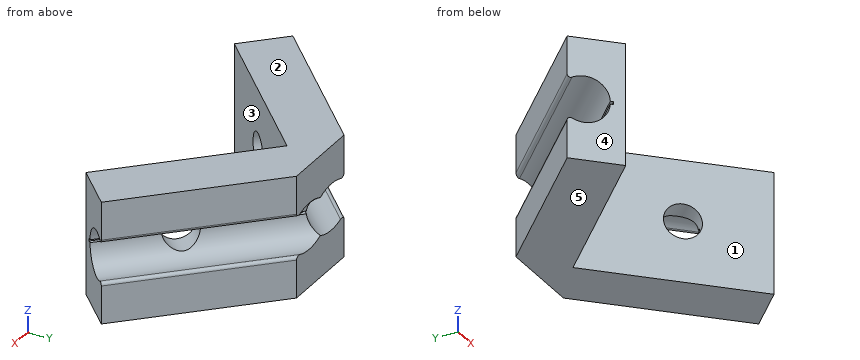
Autodesk Inventor part; units mm, degrees
ref_plane "Plano de trabajo1" through (0, 0, 0) normal (1, 0, 0) x (0, 0, -1)
ref_plane "Plano de trabajo2" through (28.2132, -15.4853, -21) normal (0.7071, 0.7071, 0) x (-0.7071, 0.7071, 0)
ref_plane "Plano de trabajo3" through (0, 0, -10.5) normal (0, 0, 1) x (1, 0, 0)
sketch "Sketch1" plane through (0, 0, 0) normal (0, 0, 1) x (1, 0, 0)
  line L0 (-7, 5.7279) -> (7, 5.7279)
  line L1 (-7, 5.7279) -> (-28.2132, -15.4853)
  line L2 (-28.2132, -15.4853) -> (-21.8492, -21.8492)
  line L3 (0, 0) -> (-21.8492, -21.8492)
  line L4 (7, 5.7279) -> (28.2132, -15.4853)
  line L5 (28.2132, -15.4853) -> (21.8492, -21.8492)
  line L6 (0, 0) -> (21.8492, -21.8492)
  line L7 (0, 15.5718) -> (0, -18.5373) construction
  dimension "d112" = 30
  dimension "d204" = 7
  dimension "d205" = 7
  dimension "d207" = 30
  dimension "d208" = 45
  dimension "d209" = 45
  dimension "d210" = 9
  dimension "d211" = 9
extrude "Extrusion1" add sketch "Sketch1" against normal blind 21
ref_plane "Plano de trabajo1" through (0, 0, 0) normal (1, 0, 0) x (0, 0, -1)
ref_plane "Plano de trabajo2" through (28.2132, -15.4853, -21) normal (0.7071, 0.7071, 0) x (-0.7071, 0.7071, 0)
sketch "Boceto2" plane through (28.2132, -15.4853, 0) normal (0.7071, -0.7071, 0) x (-0.7071, -0.7071, 0)
  line L0 (-3.8291, 10.5) -> (9.1738, 10.5) construction
  line L1 (0, 7.5) -> (0, 13.5)
  arc A0 (0, 7.5) -> (6.6379, 10.25) centre (2.6458, 10.5) ccw
  arc A1 (6.6379, 10.75) -> (0, 13.5) centre (2.6458, 10.5) ccw
  line L2 (0, 21) -> (9, 21)
  line L3 (9, 0) -> (0, 0)
  line L4 (7.1379, 10.75) -> (7.1379, 10.25)
  line L5 (7.1379, 10.25) -> (6.6379, 10.25)
  line L6 (7.1379, 10.75) -> (6.6379, 10.75)
  point P0 (0.9314, 0)
  dimension "d163" = 6
  dimension "d164" = 3
  dimension "d167" = 4
  dimension "d171" = 10.5
  dimension "d172" = 10.5
  dimension "d179" = 0.25
  dimension "d180" = 0.5
  dimension "d181" = 0.5
extrude "Extrusión2" cut sketch "Boceto2" against normal up to surface surface through (0, 0, 0) normal (1, 0, 0)
mirror "Simetría1" about plane through (0, 0, 0) normal (1, 0, 0) of "Extrusión2"
fillet "Empalme1" radius 0.5 4 edges at (17.6066, -4.8787, -7.5) (17.6066, -4.8787, -13.5) (-17.6066, -4.8787, -13.5) (-17.6066, -4.8787, -7.5)
sketch "Boceto3" plane through (28.2132, -15.4853, -21) normal (0.7071, 0.7071, 0) x (-0.7071, 0.7071, 0)
  arc A0 (30, 14.4555) -> (30.7384, 14.016) centre (30.5, 14.4555) ccw
  line L0 (30, 14.4555) -> (0, 14.4555)
  line L1 (0, 14.4555) -> (0, 14.016)
  line L2 (0, 14.016) -> (30.7384, 14.016)
  line L3 (0, 14.016) -> (30.7384, 14.016)
  line L4 (0, 10.75) -> (0, 14.016)
  arc A1 (34.9497, 13.7698) -> (30.7384, 14.016) centre (32.6458, 10.5) ccw
  line L5 (0, 10.75) -> (33.2616, 10.75)
  line L6 (0, 10.75) -> (32.7616, 10.75)
  line L7 (0, 10.75) -> (32.7616, 10.75)
  line L8 (0, 10.25) -> (0, 10.75)
  line L9 (0, 10.25) -> (32.7616, 10.25)
  line L10 (0, 10.25) -> (32.7616, 10.25)
  line L11 (0, 10.25) -> (33.2616, 10.25)
  line L12 (30.7384, 6.984) -> (0, 6.984)
  arc A2 (30.7384, 6.984) -> (34.9497, 7.2302) centre (32.6458, 10.5) ccw
  line L13 (0, 6.984) -> (0, 10.25)
  line L14 (0, 6.984) -> (0, 6.5445)
  line L15 (0, 6.5445) -> (30, 6.5445)
  arc A3 (30.7384, 6.984) -> (30, 6.5445) centre (30.5, 6.5445) ccw
  line L16 (30.7384, 6.984) -> (0, 6.984)
  line L17 (0, 6.5445) -> (30, 6.5445)
  line L18 (0, 6.5445) -> (0, 0)
  line L19 (30, 0) -> (0, 0)
  line L20 (30, 6.5445) -> (30, 0)
  line L21 (30, 14.4555) -> (0, 14.4555)
  line L22 (30, 21) -> (30, 14.4555)
  line L23 (0, 21) -> (30, 21)
  line L24 (0, 21) -> (0, 14.4555)
  circle A4 centre (14, 10.5) radius 3
  line L25 (32.7616, 10.25) -> (33.2616, 10.25)
  line L26 (32.7616, 10.25) -> (32.7616, 10.75)
  line L27 (33.2616, 10.75) -> (32.7616, 10.75)
  arc A5 (33.2616, 10.25) -> (34.9497, 7.2302) centre (37.2537, 10.5) ccw
  line L28 (0, 10.25) -> (33.2616, 10.25)
  line L29 (0, 10.75) -> (33.2616, 10.75)
  arc A6 (34.9497, 13.7698) -> (33.2616, 10.75) centre (37.2537, 10.5) ccw
  point P0 (30.8995, 21)
  dimension "d183" = 6
  dimension "d184" = 10.5
  dimension "d185" = 10.5
  dimension "d186" = 14
hole "Agujero1" at (18.3137, -5.5858, -10.5) direction (-0.7071, -0.7071, 0) diameter 6 depth 9
mirror "Simetría2" about plane through (0, 0, 0) normal (1, 0, 0) of "Agujero1"
thread "Rosca1"
thread "Rosca2"
ref_plane "Plano de trabajo3" through (0, 0, -10.5) normal (0, 0, 1) x (1, 0, 0)
properties part number "ESCUADRA UNIÓN 45 DISEÑO NUEVO V2" material "Aluminio"
CAD build for the part. Positions are in the model's coordinates, mm. Face numbers are marked on the shaded views. A direction names the side the tool comes from. Coordinates: 2 decimals unless noted, no trailing zeros. Write each loop counter-clockwise with the first axis right and the second up, starting at its lowest first coordinate (ties: lowest second). Pieces come first, ordered by that corner, then holes. Notation, with made-up numbers: M 55.5,80.5 L 67.5,80.5 A33 ccw 67.5,118.5 Z; hole C -16,26.25 d5. An arc over 180 degrees is marked long. Answer as a JSON object with one key per item and string values. Group by question number.
1) Mould opens along X. For the marked faces 3, 4 and 5 say: +X half, -X half, draft (parallel to the pull), parting line (faces both ways), or undercut.
2) Saw through at A-A (z = -11.75). Write the cut outline in (x, y), plus the area to 3 significant figures.
3) Pin check, flat tips, straight feed: pin 1 Ø3 at (x, z) = (-5, -16.5) entering from -Y; pin 2 Ø9 at (x, y) = (-19, -16.5) entering from +Z; pin 3 Ø5 at (x, z) = (11.5, -13) entering from -Y; pin 4 Ø3 at (y, z) = (-1, -6) entering from +X. Stop position of each tip, or through.
4) Saw through at B-B (z = -4). Write the cut outline in (x, y), plus the area to 3 significant figures.
5) Tool access for the marked faces 1 and 2: list every direction of +Z, -Z, +X, -X, +Y, -Y with a clear straight run to the whole face (end or side of a thin tool).
6) Wall check: line 1 (X direction, y = -18.75, z = -14.75); line 2 (X direction, y = -20, z = -13.75); line 3 (Z direction, x = 6.5, y = 0.5). Give the ranges that are in metal, low to high. Write a range as from..to.
Values follow:
{
 "1": {"face 3": "undercut", "face 4": "-X half", "face 5": "draft"},
 "2": {"outline": "M -23.66,-20.04 L -21.85,-21.85 L -13.88,-13.88 L -15.68,-12.07 Z; M -11.83,-8.21 L -10.02,-10.02 L 0,0 L 10.02,-10.02 L 11.83,-8.21 L 0,3.61 Z; M 13.88,-13.88 L 21.85,-21.85 L 23.66,-20.04 L 15.68,-12.07 Z", "area": "137 mm2"},
 "3": {"pin 1": "stops at y = -6.5", "pin 2": "stops at z = 0", "pin 3": "stops at y = -14", "pin 4": "stops at x = 15.23"},
 "4": {"outline": "M -28.21,-15.49 L -21.85,-21.85 L 0,0 L 21.85,-21.85 L 28.21,-15.49 L 7,5.73 L -7,5.73 Z", "area": "588 mm2"},
 "5": {"face 1": "+Z, -Z, -Y", "face 2": "+Z, +X, -X, +Y, -Y"},
 "6": {"line 1": "x = -24.95..-18.75, 18.75..24.95", "line 2": "x = -23.7..-20, 20..23.7", "line 3": "z = -21..-14.25, -6.75..0"}
}
